Model file for the job. Use its own axes, mm. Face numbers are marked on the shaded views. A direction names the side the tool comes from. Give positions to 0.01 mm unless a question says otherwise; leave off trailing zeros. Loops run counter-clockwise (first coordinate to the right, second up) from the corner with the lowest first, then second, coordinate; pieces in that order, holes last. Notation, with made-up numbers: M 64.5,34.5 L 74.5,34.5 A24 cw 74.5,55.5 Z; hole C -7,78.25 d9. An arc over 180 degrees is marked long. Use CSV: the item, a comma, the result in double quotes. Start each with the question number.
(1) Flat gauge pins, fed straight in: P1, Ø3, axis at x = 20.73, y = -11.97, coming from the +Z side; P2, Ø0.8, axis at x = -2, z = 1, coming from the +Y side; P3, Ø0.8, axis at x = 0, z = 0.5, coming from the -Y side (3 decimals); P4, Ø3, axis at x = 2, y = 5.5, coming from the -Z side. Where does each tip first touch, or does it go through?
(2) Slice it at B-B on y = -2. List the corners of the cut face in (x, z) (1 decimal).
(3) Slice it at C-C on z = 7. List the corners of the cut face in (x, y) (3 decimals), and give its area (3 significant figures).
(4) Tool access for the marked faces 4 and 5: list every direction of +Z, -Z, +X, -X, +Y, -Y with a clear straight run to the whole face (end or side of a thin tool).
(5) Slice it at D-D on x = -14.5. List the corners of the cut face in (y, z), and give its area (3 significant figures).
(6) Two-plate mould, pull along X, no slides. Class the marked faces 1, 2 and 3: pulls with the +X half, pulls with the -X half, needs draft (parallel to the pull), parting line crosses it, or undercut.
(7) Wall check: line 1 along Z through (x, y) = (16, -4.5); line 2 along Y through (x, z) = (7.5, 2.75); line 3 along Y through (x, z) = (11.5, 3.75). Give the ranges that are in metal, low to high. Write a range as from..to.
(8) Slice it at A-A on x = 0. List the corners of the cut face in (y, z) (1 decimal).
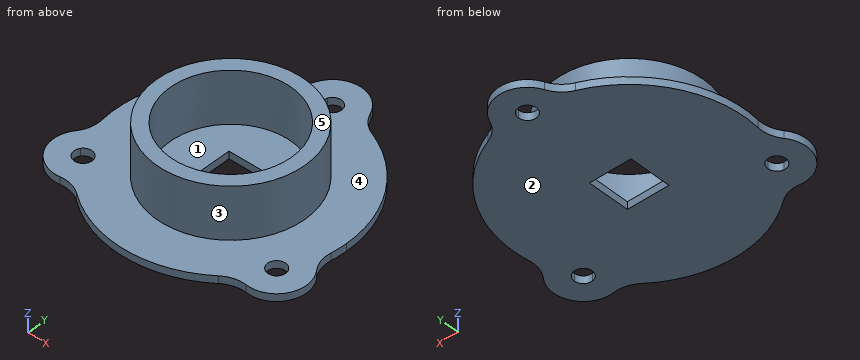
```python
from build123d import *

# Parameters (mm, degrees)
F0_R     = 15.875
F0_R_2   = 12.954
F1_DEPTH = 12.7
F0_W     = 8.89
F0_H     = 8.89
F2_DEPTH = 1.5875
F3_DEPTH = 1.5875
F4_R     = 6.35


with BuildPart() as f1:
    # F0 (on Top) → F1 (new body)
    with BuildSketch(Plane.XY):
        Circle(F0_R)
        Circle(F0_R_2, mode=Mode.SUBTRACT)
    extrude(amount=F1_DEPTH)

    # F0 (on Top) → F2 (join)
    with BuildSketch(Plane.XY):
        Circle(F0_R_2)
        Rectangle(F0_W, F0_H, mode=Mode.SUBTRACT)
    extrude(amount=F2_DEPTH)

    # F0 (on Top) → F3 (join)
    with BuildSketch(Plane.XY):
        with BuildLine():
            ThreePointArc((23.9050999455, -6.4692674698), (24.5490837421, -3.2630832697), (24.765, 0))
            ThreePointArc((24.765, 0), (19.6285885254, 15.1004548773), (6.35, 23.9370575677))
            ThreePointArc((6.35, 23.9370575677), (4.0651088886, 24.4290833787), (1.7440091422, 24.703515076))
            ThreePointArc((1.7440091422, 24.703515076), (1.8643178935, 24.3286489263), (1.905, 23.9370575677))
            ThreePointArc((1.905, 23.9370575677), (-0.3915913586, 22.0727396742), (-1.7440091422, 24.703515076))
            ThreePointArc((-1.7440091422, 24.703515076), (-4.0651088886, 24.4290833787), (-6.35, 23.9370575677))
            ThreePointArc((-6.35, 23.9370575677), (-21.4471191247, 12.3825), (-23.9050999455, -6.4692674698))
            ThreePointArc((-23.9050999455, -6.4692674698), (-23.1887612414, -8.6940541227), (-22.2658761897, -10.8414013165))
            ThreePointArc((-22.2658761897, -10.8414013165), (-20.1370690632, -10.1581864481), (-18.8250999455, -11.9685287839))
            ThreePointArc((-18.8250999455, -11.9685287839), (-19.3113489683, -13.239815795), (-20.5218670475, -13.8621137596))
            ThreePointArc((-20.5218670475, -13.8621137596), (-19.1236523528, -15.735029256), (-17.5550999455, -17.4677900979))
            ThreePointArc((-17.5550999455, -17.4677900979), (0, -24.765), (17.5550999455, -17.4677900979))
            ThreePointArc((17.5550999455, -17.4677900979), (19.1236523528, -15.735029256), (20.5218670475, -13.8621137596))
            ThreePointArc((20.5218670475, -13.8621137596), (19.0803215513, -11.0160287839), (22.2658761897, -10.8414013165))
            ThreePointArc((22.2658761897, -10.8414013165), (23.1887612414, -8.6940541227), (23.9050999455, -6.4692674698))
        make_face()
        Circle(F0_R, mode=Mode.SUBTRACT)
        with BuildLine():
            ThreePointArc((1.7440091422, 24.703515076), (4.0651088886, 24.4290833787), (6.35, 23.9370575677))
            ThreePointArc((6.35, 23.9370575677), (0, 30.2870575677), (-6.35, 23.9370575677))
            ThreePointArc((-6.35, 23.9370575677), (-4.0651088886, 24.4290833787), (-1.7440091422, 24.703515076))
            ThreePointArc((-1.7440091422, 24.703515076), (0, 25.8420575677), (1.7440091422, 24.703515076))
        make_face()
        with BuildLine():
            ThreePointArc((17.5550999455, -17.4677900979), (26.2293612595, -15.1435287839), (23.9050999455, -6.4692674698))
            ThreePointArc((23.9050999455, -6.4692674698), (23.1887612414, -8.6940541227), (22.2658761897, -10.8414013165))
            ThreePointArc((22.2658761897, -10.8414013165), (22.5404422812, -11.3754979015), (22.6350999455, -11.9685287839))
            ThreePointArc((22.6350999455, -11.9685287839), (22.0013869566, -13.3872797611), (20.5218670475, -13.8621137596))
            ThreePointArc((20.5218670475, -13.8621137596), (19.1236523528, -15.735029256), (17.5550999455, -17.4677900979))
        make_face()
        with BuildLine():
            ThreePointArc((-22.2658761897, -10.8414013165), (-23.1887612414, -8.6940541227), (-23.9050999455, -6.4692674698))
            ThreePointArc((-23.9050999455, -6.4692674698), (-26.2293612595, -15.1435287839), (-17.5550999455, -17.4677900979))
            ThreePointArc((-17.5550999455, -17.4677900979), (-19.1236523528, -15.735029256), (-20.5218670475, -13.8621137596))
            ThreePointArc((-20.5218670475, -13.8621137596), (-22.3798783397, -12.9210287839), (-22.2658761897, -10.8414013165))
        make_face()
    extrude(amount=F3_DEPTH)

    # F4
    f4_edges = [f1.edges().sort_by_distance(p)[0] for p in [
        (-23.9051, -6.469267, 0.79375),
        (17.5551, -17.46779, 0.79375),
        (6.35, 23.937058, 0.79375),
        (23.9051, -6.469267, 0.79375),
        (-6.35, 23.937058, 0.79375),
        (-17.5551, -17.46779, 0.79375),
    ]]
    fillet(f4_edges, radius=F4_R)


solid = f1.part
```
Reply:
1,P1,"passes through"
1,P2,"stops at y = 30.08"
1,P3,"stops at y = -24.765"
1,P4,"stops at z = 0"
2,outline,"M -24.7,0 L -4.4,0 L -4.4,1.6 L -12.8,1.6 L -12.8,12.7 L -15.7,12.7 L -15.7,1.6 L -24.7,1.6 Z; M 4.4,0 L 24.7,0 L 24.7,1.6 L 15.7,1.6 L 15.7,12.7 L 12.8,12.7 L 12.8,1.6 L 4.4,1.6 Z"
3,outline,"C 0,0 d31.75; hole C 0,0 d25.908"
3,area,"265 mm^2"
4,face 4,"+Z"
4,face 5,"+Z, +X, -X, +Y, -Y"
5,outline,"M -20.08,0 L 20.08,0 L 20.08,1.59 L 6.46,1.59 L 6.46,12.7 L -6.46,12.7 L -6.46,1.59 L -20.08,1.59 Z"
5,area,"207 mm^2"
6,face 1,"undercut"
6,face 2,"needs draft"
6,face 3,"parting line crosses it"
7,line 1,"z = 0..1.59"
7,line 2,"y = -13.99..-10.56, 10.56..13.99"
7,line 3,"y = -10.94..-5.96, 5.96..10.94"
8,outline,"M -24.8,0 L -4.4,0 L -4.4,1.6 L -13,1.6 L -13,12.7 L -15.9,12.7 L -15.9,1.6 L -24.8,1.6 Z; M 4.4,0 L 22,0 L 22,1.6 L 15.9,1.6 L 15.9,12.7 L 13,12.7 L 13,1.6 L 4.4,1.6 Z; M 25.8,0 L 30.3,0 L 30.3,1.6 L 25.8,1.6 Z"
